```python
from build123d import *

# Parameters (mm, degrees)
SKETCH1_R           = 6.39375
BOSS_EXTRUDE1_DEPTH = 4.2
BOSS_EXTRUDE2_DEPTH = 3
FILLET1_R           = 1
SKETCH3_R           = 1.5
CUT_EXTRUDE1_DEPTH  = 17.968242557
BOSS_EXTRUDE3_DEPTH = 3
CHAMFER1_SIZE       = 6
CHAMFER2_SIZE       = 9
SKETCH6_W           = 5
SKETCH6_H           = 3
BOSS_EXTRUDE4_DEPTH = 2


with BuildPart() as part:
    # Sketch1 → Boss-Extrude1 (new body)
    with BuildSketch(Plane(origin=(0, 0, 0), x_dir=(1, 0, 0), z_dir=(0, 1, 0))):
        with Locations(Location((0, 0, 0), (0, 0, 270))):
            Circle(SKETCH1_R)
    extrude(amount=BOSS_EXTRUDE1_DEPTH)

    # Sketch2 → Boss-Extrude2 (add)
    with BuildSketch(Plane(origin=(0, 0, 0), x_dir=(1, 0, 0), z_dir=(0, 1, 0))):
        with BuildLine():
            Line((-1.433648629, 6.23094621), (-1.959549626, 8.516625387))
            add(Edge.make_bspline(
                [(-1.959549626, 8.516625387), (-1.745269759, 9.644412797), (-1.223586565, 10.731441367), (-0.488991141, 11.614711045)],
                knots=[0, 0, 0, 0, 1, 1, 1, 1], degree=3))
            ThreePointArc((-0.488991141, 11.614711045), (0, 11.625), (0.488991141, 11.614711045))
            add(Edge.make_bspline(
                [(1.959549626, 8.516625387), (1.745269759, 9.644412797), (1.223586565, 10.731441367), (0.488991141, 11.614711045)],
                knots=[0, 0, 0, 0, 1, 1, 1, 1], degree=3))
            Line((1.959549626, 8.516625387), (1.433648629, 6.23094621))
            ThreePointArc((1.433648629, 6.23094621), (0, 6.39375), (-1.433648629, 6.23094621))
        make_face()
        with BuildLine():
            Line((3.392201651, 5.419686986), (4.636552736, 7.407774392))
            add(Edge.make_bspline(
                [(4.636552736, 7.407774392), (5.585537608, 8.053721771), (6.723068605, 8.45348132), (7.86707199, 8.558609894)],
                knots=[0, 0, 0, 0, 1, 1, 1, 1], degree=3))
            ThreePointArc((7.86707199, 8.558609894), (8.220116331, 8.220116331), (8.558609894, 7.86707199))
            add(Edge.make_bspline(
                [(7.407774392, 4.636552736), (8.053721771, 5.585537608), (8.45348132, 6.723068605), (8.558609894, 7.86707199)],
                knots=[0, 0, 0, 0, 1, 1, 1, 1], degree=3))
            Line((7.407774392, 4.636552736), (5.419686986, 3.392201651))
            ThreePointArc((5.419686986, 3.392201651), (4.521063982, 4.521063982), (3.392201651, 5.419686986))
        make_face()
        with BuildLine():
            Line((6.23094621, 1.433648629), (8.516625387, 1.959549626))
            add(Edge.make_bspline(
                [(8.516625387, 1.959549626), (9.644412797, 1.745269759), (10.731441367, 1.223586565), (11.614711045, 0.488991141)],
                knots=[0, 0, 0, 0, 1, 1, 1, 1], degree=3))
            ThreePointArc((11.614711045, 0.488991141), (11.625, 0), (11.614711045, -0.488991141))
            add(Edge.make_bspline(
                [(8.516625387, -1.959549626), (9.644412797, -1.745269759), (10.731441367, -1.223586565), (11.614711045, -0.488991141)],
                knots=[0, 0, 0, 0, 1, 1, 1, 1], degree=3))
            Line((8.516625387, -1.959549626), (6.23094621, -1.433648629))
            ThreePointArc((6.23094621, -1.433648629), (6.39375, 0), (6.23094621, 1.433648629))
        make_face()
        with BuildLine():
            Line((5.419686986, -3.392201651), (7.407774392, -4.636552736))
            add(Edge.make_bspline(
                [(7.407774392, -4.636552736), (8.053721771, -5.585537608), (8.45348132, -6.723068605), (8.558609894, -7.86707199)],
                knots=[0, 0, 0, 0, 1, 1, 1, 1], degree=3))
            ThreePointArc((8.558609894, -7.86707199), (8.220116331, -8.220116331), (7.86707199, -8.558609894))
            add(Edge.make_bspline(
                [(4.636552736, -7.407774392), (5.585537608, -8.053721771), (6.723068605, -8.45348132), (7.86707199, -8.558609894)],
                knots=[0, 0, 0, 0, 1, 1, 1, 1], degree=3))
            Line((4.636552736, -7.407774392), (3.392201651, -5.419686986))
            ThreePointArc((3.392201651, -5.419686986), (4.521063982, -4.521063982), (5.419686986, -3.392201651))
        make_face()
        with BuildLine():
            Line((1.433648629, -6.23094621), (1.959549626, -8.516625387))
            add(Edge.make_bspline(
                [(1.959549626, -8.516625387), (1.745269759, -9.644412797), (1.223586565, -10.731441367), (0.488991141, -11.614711045)],
                knots=[0, 0, 0, 0, 1, 1, 1, 1], degree=3))
            ThreePointArc((0.488991141, -11.614711045), (0, -11.625), (-0.488991141, -11.614711045))
            add(Edge.make_bspline(
                [(-1.959549626, -8.516625387), (-1.745269759, -9.644412797), (-1.223586565, -10.731441367), (-0.488991141, -11.614711045)],
                knots=[0, 0, 0, 0, 1, 1, 1, 1], degree=3))
            Line((-1.959549626, -8.516625387), (-1.433648629, -6.23094621))
            ThreePointArc((-1.433648629, -6.23094621), (0, -6.39375), (1.433648629, -6.23094621))
        make_face()
        with BuildLine():
            Line((-3.392201651, -5.419686986), (-4.636552736, -7.407774392))
            add(Edge.make_bspline(
                [(-4.636552736, -7.407774392), (-5.585537608, -8.053721771), (-6.723068605, -8.45348132), (-7.86707199, -8.558609894)],
                knots=[0, 0, 0, 0, 1, 1, 1, 1], degree=3))
            ThreePointArc((-7.86707199, -8.558609894), (-8.220116331, -8.220116331), (-8.558609894, -7.86707199))
            add(Edge.make_bspline(
                [(-7.407774392, -4.636552736), (-8.053721771, -5.585537608), (-8.45348132, -6.723068605), (-8.558609894, -7.86707199)],
                knots=[0, 0, 0, 0, 1, 1, 1, 1], degree=3))
            Line((-7.407774392, -4.636552736), (-5.419686986, -3.392201651))
            ThreePointArc((-5.419686986, -3.392201651), (-4.521063982, -4.521063982), (-3.392201651, -5.419686986))
        make_face()
        with BuildLine():
            Line((-6.23094621, -1.433648629), (-8.516625387, -1.959549626))
            add(Edge.make_bspline(
                [(-8.516625387, -1.959549626), (-9.644412797, -1.745269759), (-10.731441367, -1.223586565), (-11.614711045, -0.488991141)],
                knots=[0, 0, 0, 0, 1, 1, 1, 1], degree=3))
            ThreePointArc((-11.614711045, -0.488991141), (-11.625, 0), (-11.614711045, 0.488991141))
            add(Edge.make_bspline(
                [(-8.516625387, 1.959549626), (-9.644412797, 1.745269759), (-10.731441367, 1.223586565), (-11.614711045, 0.488991141)],
                knots=[0, 0, 0, 0, 1, 1, 1, 1], degree=3))
            Line((-8.516625387, 1.959549626), (-6.23094621, 1.433648629))
            ThreePointArc((-6.23094621, 1.433648629), (-6.39375, 0), (-6.23094621, -1.433648629))
        make_face()
        with BuildLine():
            Line((-5.419686986, 3.392201651), (-7.407774392, 4.636552736))
            add(Edge.make_bspline(
                [(-7.407774392, 4.636552736), (-8.053721771, 5.585537608), (-8.45348132, 6.723068605), (-8.558609894, 7.86707199)],
                knots=[0, 0, 0, 0, 1, 1, 1, 1], degree=3))
            ThreePointArc((-8.558609894, 7.86707199), (-8.220116331, 8.220116331), (-7.86707199, 8.558609894))
            add(Edge.make_bspline(
                [(-4.636552736, 7.407774392), (-5.585537608, 8.053721771), (-6.723068605, 8.45348132), (-7.86707199, 8.558609894)],
                knots=[0, 0, 0, 0, 1, 1, 1, 1], degree=3))
            Line((-4.636552736, 7.407774392), (-3.392201651, 5.419686986))
            ThreePointArc((-3.392201651, 5.419686986), (-4.521063982, 4.521063982), (-5.419686986, 3.392201651))
        make_face()
    extrude(amount=BOSS_EXTRUDE2_DEPTH)

    # Fillet1
    fillet1_edges = [part.edges().sort_by_distance(p)[0] for p in [
        (-5.419686986, 1.5, -3.392201651),
        (-3.392201651, 1.5, -5.419686986),
        (3.392201651, 1.5, -5.419686986),
        (5.419686986, 1.5, -3.392201651),
        (6.23094621, 1.5, -1.433648629),
        (6.23094621, 1.5, 1.433648629),
        (5.419686986, 1.5, 3.392201651),
        (3.392201651, 1.5, 5.419686986),
        (1.433648629, 1.5, 6.23094621),
        (-1.433648629, 1.5, 6.23094621),
        (-3.392201651, 1.5, 5.419686986),
        (-5.419686986, 1.5, 3.392201651),
        (-1.433648629, 1.5, -6.23094621),
        (1.433648629, 1.5, -6.23094621),
        (-6.23094621, 1.5, 1.433648629),
        (-6.23094621, 1.5, -1.433648629),
    ]]
    fillet(fillet1_edges, radius=FILLET1_R)

    # Sketch3 → Cut-Extrude1 (cut, through all)
    with BuildSketch(Plane(origin=(0, 4.2, 0), x_dir=(1, 0, 0), z_dir=(0, 1, 0))):
        with Locations(Location((0, 0, 0), (0, 0, 270))):
            Circle(SKETCH3_R)
    extrude(amount=-CUT_EXTRUDE1_DEPTH, mode=Mode.SUBTRACT)

    # Sketch5 → Boss-Extrude3 (add)
    with BuildSketch(Plane.XZ):
        Polygon((-3.2, 4), (3.2, 4), (3.2, 34), (-9.3, 34), (-9.3, 27.6), (-3.2, 27.6), align=None)
    extrude(amount=-BOSS_EXTRUDE3_DEPTH)

    # Chamfer1
    chamfer1_edges = [part.edges().sort_by_distance(p)[0] for p in [
        (-3.2, 1.5, 27.6),
    ]]
    chamfer(chamfer1_edges, length=CHAMFER1_SIZE)

    # Chamfer2
    chamfer2_edges = [part.edges().sort_by_distance(p)[0] for p in [
        (3.2, 1.5, 34),
    ]]
    chamfer(chamfer2_edges, length=CHAMFER2_SIZE)

    # Sketch6 → Boss-Extrude4 (add)
    with BuildSketch(Plane.XZ):
        with Locations((0, -5)):
            Rectangle(SKETCH6_W, SKETCH6_H)
        with Locations((0, 5)):
            Rectangle(SKETCH6_W, SKETCH6_H)
    extrude(amount=BOSS_EXTRUDE4_DEPTH)


solid = part.part
```
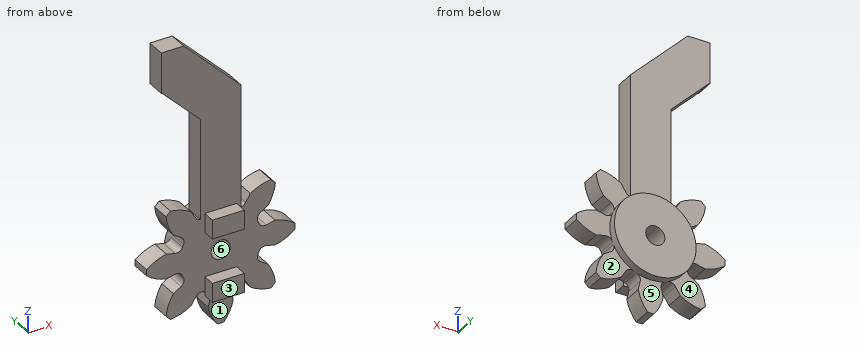
Can you work these out from the model? Positions are in its coordinate system, mm. Face numbers are marked on the shaded views. A direction names the side the tool comes from. Round coordinates to 2 decimals unless told otherwise and drop trailing zeros. Loops run counter-clockwise (first coordinate to the right, second up) from the corner with the lowest first, then second, coordinate; pieces in that order, holes last.
Item 1: Please list where these lines run through material, in increasing order: L1, parallel to X at y = 2.85, z = 0 (3 decimals); L2, parallel to X at y = -1.5, z = -4.5; L3, parallel to X at y = 1.25, z = -6.5.
Item 2: Suppose I cut it at C-C, the plane z = 0. Write out the boundary of the cut face in (x, y) (3 decimals), then the cut area to 3 significant figures.
Item 3: Suppose I cut it at A-A, the plane x = 0. Write out the boundary of the cut face in (y, z) (3 decimals).
Item 4: Suppose I cut it at B-B, the plane y = -1.5. Write out the boundary of the cut face in (x, z), then the cut area to 3 significant figures.
Item 5: If we mould it in two halves opening along Z, with no side actions, what happens to the marked faces 5 and 6? For each: +Z half, -Z half, draft (parallel to the pull), parting line (faces both ways), or undercut.
Item 6: Which directions (+Z, -Z, +X, -X, +Y, -Y) give clear straight access to the entire face, cutting with the end or side of a thin tool? Please do the marked faces 1, 2, 3 and 4.
Item 7: Suppose I cut it at D-D, the plane z = 24. Write out the boundary of the cut face in (x, y).
Item 8: Will these pins go through, and if not, where does the flat tip stop? pin 1 Ø3.5 at (y, z) = (2, 29.5) entering from -X; pin 2 Ø4.5 at (x, z) = (-4.5, -6.5) entering from +Y; pin 3 Ø11.5 at (x, z) = (2, 17.5) entering from -Y; pin 4 Ø0.6 at (y, z) = (-1.5, -5) entering from +X.
Reported:
1. L1: x = -11.625 to -1.5, 1.5 to 11.625
1. L2: x = -2.5 to 2.5
1. L3: x = -8.29 to -4.07, -1.71 to 1.71, 4.07 to 8.29
2. outline: (-11.625, 0) - (-1.5, 0) - (-1.5, 4.2) - (-6.394, 4.2) - (-6.394, 3) - (-11.625, 3) - close; (1.5, 0) - (11.625, 0) - (11.625, 3) - (6.394, 3) - (6.394, 4.2) - (1.5, 4.2) - close
2. area: 72.5 mm2
3. outline: (-2, -6.5) - (0, -6.5) - (0, -11.625) - (3, -11.625) - (3, -6.394) - (4.2, -6.394) - (4.2, -1.5) - (0, -1.5) - (0, -3.5) - (-2, -3.5) - close; (-2, 3.5) - (0, 3.5) - (0, 1.5) - (4.2, 1.5) - (4.2, 6.394) - (3, 6.394) - (3, 28.2) - (0, 28.2) - (0, 6.5) - (-2, 6.5) - close
4. outline: (-2.5, -6.5) - (2.5, -6.5) - (2.5, -3.5) - (-2.5, -3.5) - close; (-2.5, 3.5) - (2.5, 3.5) - (2.5, 6.5) - (-2.5, 6.5) - close
4. area: 30.0 mm2
5. face 5: draft
5. face 6: undercut
6. face 1: -Z, +X, -X, -Y
6. face 2: -Z, +X, +Y
6. face 3: +Z, -Z, +X, -X, -Y
6. face 4: -Z, -X, +Y
7. outline: (-5.6, 0) - (3.2, 0) - (3.2, 3) - (-5.6, 3) - close
8. pin 1: stops at x = -9.3
8. pin 2: stops at y = 4.2
8. pin 3: stops at y = 0
8. pin 4: stops at x = 2.5
